Geometry check sheet. Reference: the model listing, model coordinates, mm. Give positions to 0.01 mm unless a question says otherwise; leave off trailing zeros. Loops run counter-clockwise (first coordinate to the right, second up) from the corner with the lowest first, then second, coordinate; pieces in that order, holes last. Notation, with made-up numbers: (75.5, 6.5) -> (117.5, 6.5) arc R33 ccw to (117.5, 37.5) -> close; hole circle Ø5 at (-7, 44). An arc over 180 degrees is marked (long way). Answer in a Markdown table with one row per item. Add a question column.
```python
from build123d import *

# Parameters (mm, degrees)
SKETCH2_W           = 251.86
SKETCH2_H           = 251.86
BOSS_EXTRUDE1_DEPTH = 24
BOSS_EXTRUDE1_DRAFT = -2
SHELL1_T            = -2
CUT_EXTRUDE1_START  = -10
SKETCH3_R           = 1.7
CUT_EXTRUDE1_DEPTH  = 294.998422143
SKETCH4_R           = 1.7
CUT_EXTRUDE2_DEPTH  = 10


with BuildPart() as part:
    # Sketch2 → Boss-Extrude1 (with draft: the straight prism first)
    with BuildSketch(Plane(origin=(0, 0, 0), x_dir=(1, 0, 0), z_dir=(0, 1, 0))):
        Rectangle(SKETCH2_W, SKETCH2_H)
    extrude(amount=BOSS_EXTRUDE1_DEPTH)
    # Boss-Extrude1: the draft: its side faces are tilted about the plane it starts from
    boss_extrude1_sides = [part.faces().sort_by_distance(p)[0] for p in [
        (0, 12, 125.93),
        (125.93, 12, 0),
        (0, 12, -125.93),
        (-125.93, 12, 0),
    ]]
    draft(boss_extrude1_sides, Plane(origin=(0, 0, 0), x_dir=(1, 0, 0), z_dir=(0, 1, 0)), BOSS_EXTRUDE1_DRAFT)

    # Shell1
    shell1_openings = [part.faces().sort_by_distance(p)[0] for p in [
        (0, 24, 0),
        (0, 0, 0),
    ]]
    offset(amount=SHELL1_T, openings=shell1_openings, kind=Kind.INTERSECTION)

    # Sketch3 → Cut-Extrude1 (cut)
    with BuildSketch(Plane(origin=(-125.776620425, -4.392216369, 0), x_dir=(0, 0, 1), z_dir=(-0.9993908270190958, -0.03489949670250105, 0)).offset(CUT_EXTRUDE1_START)):
        with Locations(Location((-95, 20.409522683, 0), (0, 0, 270))):
            Circle(SKETCH3_R)
        with Locations(Location((0, 20.409522683, 0), (0, 0, 270))):
            Circle(SKETCH3_R)
        with Locations(Location((95, 20.409522683, 0), (0, 0, 270))):
            Circle(SKETCH3_R)
    cut_extrude1 = extrude(amount=CUT_EXTRUDE1_DEPTH, mode=Mode.SUBTRACT)

    # Mirror1: Cut-Extrude1 across plane
    add(cut_extrude1.mirror(Plane(origin=(0, 0, 0), x_dir=(0, 0, 1), z_dir=(1, 0, 0))), mode=Mode.SUBTRACT)

    # Sketch4 → Cut-Extrude2 (cut)
    with BuildSketch(Plane(origin=(0, -4.392216369, -125.776620425), x_dir=(-1, 0, 0), z_dir=(0, -0.03489949670250105, -0.9993908270190958))):
        with Locations(Location((-95, 20.409522683, 0), (0, 0, 90))):
            Circle(SKETCH4_R)
        with Locations(Location((0, 20.409522683, 0), (0, 0, 90))):
            Circle(SKETCH4_R)
        with Locations(Location((95, 20.409522683, 0), (0, 0, 90))):
            Circle(SKETCH4_R)
    cut_extrude2 = extrude(amount=-CUT_EXTRUDE2_DEPTH, mode=Mode.SUBTRACT)

    # Mirror2: Cut-Extrude2 across plane
    add(cut_extrude2.mirror(Plane.XY), mode=Mode.SUBTRACT)


solid = part.part
```
1. Sectioned sample at A-A (x = 27). Enter the section's corners in (y, z).
2. Sectioned sample at B-B (z = 85.5). Enter the section's corners in (x, y).
3. Sectioned sample at C-C (y = 10.25). Enter the section's corners in (x, z), plus the area to 3 significant figures.
4. Gauge pin test, flat ends, axial feed: pin 1 Ø1.5 at (y, z) = (11.5, -93) entering from +X; pin 2 Ø5 at (y, z) = (18, -63) entering from +X; pin 3 Ø3 at (y, z) = (10.5, 11) entering from -X. Record the tip position at first contact, or that the pin passes through.
5. Material ranges on L1, parallel to Z at x = -2, y = 2; L2, parallel to X at y = 1.25, z = 89.5; L3, parallel to Z at x = -43.5, y = 22.25, recorded low to high. Write a range as from..to.
Response:
| question | item | result |
|---|---|---|
| 1 | outline | (0, -125.93) -> (24, -126.77) -> (24, -124.77) -> (0, -123.93) -> close; (0, 123.93) -> (24, 124.77) -> (24, 126.77) -> (0, 125.93) -> close |
| 2 | outline | (-126.77, 24) -> (-125.93, 0) -> (-123.93, 0) -> (-124.77, 24) -> close; (123.93, 0) -> (125.93, 0) -> (126.77, 24) -> (124.77, 24) -> close |
| 3 | outline | (-126.29, -126.29) -> (126.29, -126.29) -> (126.29, 126.29) -> (-126.29, 126.29) -> close; hole (-124.29, -124.29) -> (124.29, -124.29) -> (124.29, 124.29) -> (-124.29, 124.29) -> close |
| 3 | area | 2,010 mm2 |
| 4 | pin 1 | stops at x = 126.36 |
| 4 | pin 2 | stops at x = 126.65 |
| 4 | pin 3 | stops at x = -126.35 |
| 5 | L1 | z = -126..-124, 124..126 |
| 5 | L2 | x = -125.97..-123.97, 123.97..125.97 |
| 5 | L3 | z = -126.71..-124.71, 124.71..126.71 |
